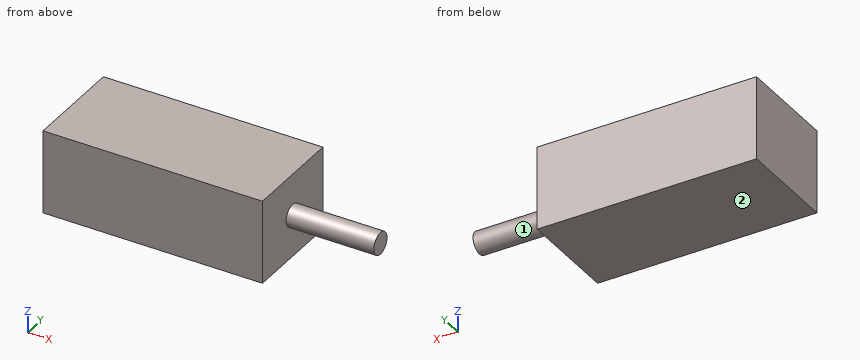
from build123d import *

# Parameters (mm, degrees)
SKETCH1_R           = 1.25
BOSS_EXTRUDE1_DEPTH = 10
SKETCH2_W           = 9.5
SKETCH2_H           = 11.5
BOSS_EXTRUDE2_DEPTH = 25


with BuildPart() as part:
    # Sketch1 → Boss-Extrude1 (new body)
    with BuildSketch(Plane(origin=(0, 0, 0), x_dir=(0, 0, -1), z_dir=(1, 0, 0))):
        Circle(SKETCH1_R)
    extrude(amount=BOSS_EXTRUDE1_DEPTH)

    # Sketch2 → Boss-Extrude2 (add)
    with BuildSketch(Plane.ZY):
        Rectangle(SKETCH2_W, SKETCH2_H)
    extrude(amount=BOSS_EXTRUDE2_DEPTH)


solid = part.part
Read the model definition and answer for the solid it produces. Units are mm, in the model's axes. Face numbers are marked on the shaded views. A direction names the side the tool comes from. Give positions to 0.01 mm unless a question says otherwise; leave off trailing zeros. Write each loop counter-clockwise with the first axis right and the second up, starting at its lowest first coordinate (ties: lowest second). Pieces come first, ordered by that corner, then holes. Notation, with made-up numbers: (13, -5.5) - (72, -5.5) arc R24 cw to (72, 31.5) - close; hole circle Ø3 at (-39.5, 41). An arc over 180 degrees is marked (long way). Return JSON: item names as keys, results as strings.
Q1. A cutting plane is placed at A-A, the plane y = 0. Determine the outline of the cut face in (x, z).
Reply:
{"outline": "(-25, -4.75) - (0, -4.75) - (0, -1.25) - (10, -1.25) - (10, 1.25) - (0, 1.25) - (0, 4.75) - (-25, 4.75) - close"}
Q2. A cutting plane is placed at B-B, the plane z = 0. Determine the outline of the cut face in (x, y).
Reply:
{"outline": "(-25, -5.75) - (0, -5.75) - (0, -1.25) - (10, -1.25) - (10, 1.25) - (0, 1.25) - (0, 5.75) - (-25, 5.75) - close"}
Q3. A cutting plane is placed at C-C, the plane y = -5. Determine the outline of the cut face in (x, z).
Reply:
{"outline": "(-25, -4.75) - (0, -4.75) - (0, 4.75) - (-25, 4.75) - close"}
Q4. For the marked faces 1 and 2, determine the directions among +Z, -Z, +X, -X, +Y, -Y from which every point of the face is accessible in a straight line to the end or side of a thin tool.
Reply:
{"face 1": "+X", "face 2": "-Z, +X, -X, +Y, -Y"}
Q5. A cutting plane is placed at D-D, the plane z = 2. Determine the outline of the cut face in (x, y).
Reply:
{"outline": "(-25, -5.75) - (0, -5.75) - (0, 5.75) - (-25, 5.75) - close"}
Q6. Consider line 1 along X through (y, z) = (0, -3); line 2 along Z through (x, y) = (8, 1). Determine where each line is inside the solid, lowest interval first. Write a range as [from, to].
Reply:
{"line 1": "[-25, 0]", "line 2": "[-0.75, 0.75]"}
